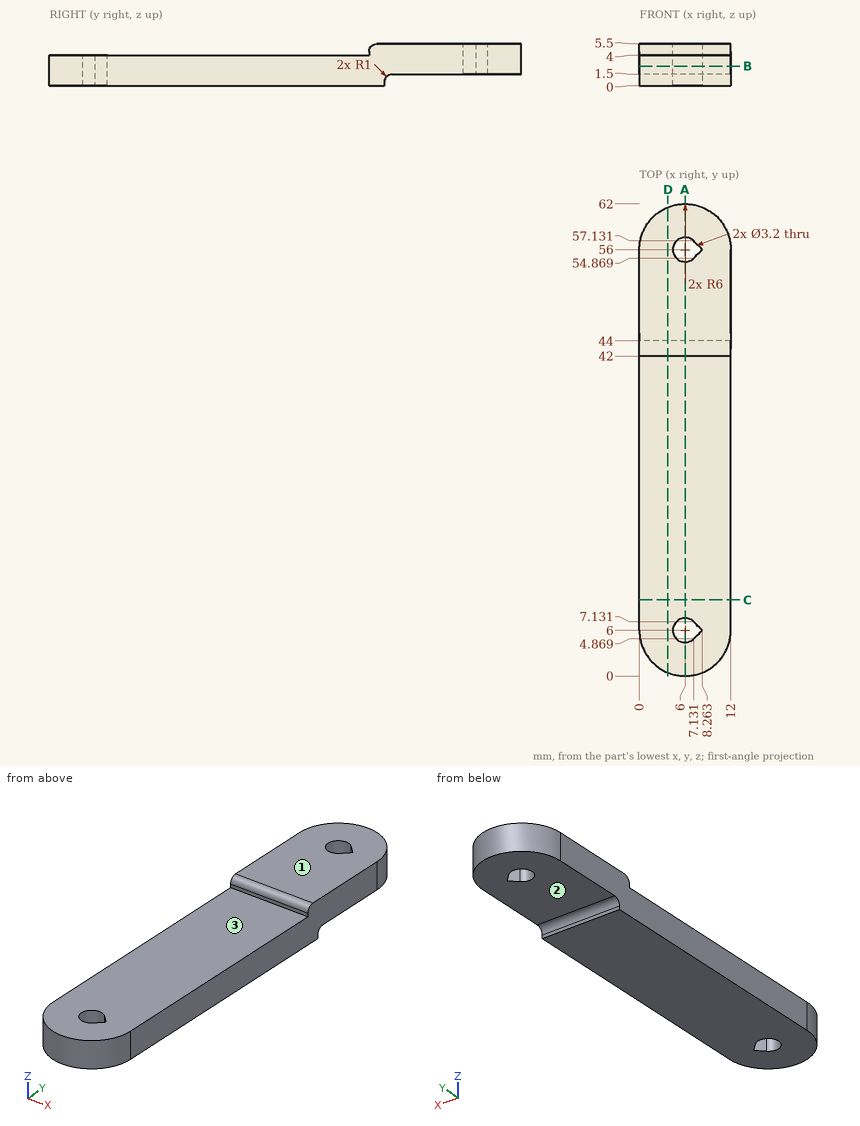
The figure shows three views and two pictorial views of one solid part (mm, origin at its lowest corner). Answer the questions. A direction names the side the tool comes from. Round coordinates to 2 decimals unless told otherwise and drop trailing zeros. Loops run counter-clockwise (first coordinate to the right, second up) from the corner with the lowest first, then second, coordinate; pieces in that order, holes last. Notation, with made-up numbers: (-8.5, -24) -> (-3.5, -24) arc R13 cw to (-3.5, -20) -> close; hole circle Ø5 at (40, 47). An arc over 180 degrees is marked (long way). Use one line per item in the form item = value.
(1) Find section C-C on y = 10. Give the vertices of the cut face in (x, z).
Answer list:
outline = (0, 0) -> (12, 0) -> (12, 4) -> (0, 4) -> close
(2) Flat-ended cylindrical pins translate along their axes: P1, Ø2, axis at x = 4, y = 27, coming from the +Z side; P2, Ø2, axis at x = 10.5, z = 3.5, coming from the -Y side; P3, Ø2, axis at x = 8, z = 2.5, coming from the -Y side; P4, Ø4, axis at x = 6, y = 56, coming from the +Z side. Find the tip coordinate at first contact, or state that the pin passes through.
Answer list:
P1 = 4
P2 = 1.13
P3 = 0.08
P4 = 5.5
(3) Find section B-B on z = 2.6. Give the vertices of the cut face in (x, y), then the cut area to 3 significant figures.
Answer list:
outline = (0, 6) arc R6 ccw to (12, 6) -> (12, 56) arc R6 ccw to (0, 56) -> close; hole (7.13, 4.87) -> (8.26, 6) -> (7.13, 7.13) arc R1.6 ccw (long way) to start; hole (7.13, 54.87) -> (8.26, 56) -> (7.13, 57.13) arc R1.6 ccw (long way) to start
area = 696 mm2
(4) A tool of negligible diameter and unlimited length cuts with its end or side. For the marked faces 1, 2 and 3, from which of +Z, -Z, +X, -X, +Y, -Y can it reach the whole face along a straight path? Write none if from no direction.
Answer list:
face_1 = +Z, +X, -X, +Y, -Y
face_2 = -Z, +X, -X, +Y
face_3 = +Z, +X, -X, -Y
(5) Find section D-D on x = 3.75. Give the vertices of the cut face in (y, z).
Answer list:
outline = (0.44, 0) -> (44, 0) -> (44, 0.5) arc R1 cw to (45, 1.5) -> (61.56, 1.5) -> (61.56, 5.5) -> (43, 5.5) arc R1 ccw to (42, 4.5) -> (42, 4) -> (0.44, 4) -> close
(6) Find section A-A on x = 6. Give the vertices of the cut face in (y, z).
Answer list:
outline = (0, 0) -> (4.4, 0) -> (4.4, 4) -> (0, 4) -> close; (7.6, 0) -> (44, 0) -> (44, 0.5) arc R1 cw to (45, 1.5) -> (54.4, 1.5) -> (54.4, 5.5) -> (43, 5.5) arc R1 ccw to (42, 4.5) -> (42, 4) -> (7.6, 4) -> close; (57.6, 1.5) -> (62, 1.5) -> (62, 5.5) -> (57.6, 5.5) -> close
(7) Straight lines are drawn through the part: line 1 (Y direction, x = 6, z = 1.6); line 2 (Y direction, x = 5.25, z = 2.2); line 3 (Z direction, x = 6, y = 20.5). For each, find the intervals that lie inside material, in ascending order.
Answer list:
line_1 = 0 to 4.4, 7.6 to 54.4, 57.6 to 62
line_2 = 0.05 to 4.59, 7.41 to 54.59, 57.41 to 61.95
line_3 = 0 to 4
